Source: CAD feature listing. Evaluate the final solid. Frame: model axes, mm. Give positions to 0.01 mm unless a question says otherwise; leave off trailing zeros. Loops run counter-clockwise (first coordinate to the right, second up) from the corner with the lowest first, then second, coordinate; pieces in that order, holes last. Notation, with made-up numbers: M 39.25,9 L 58.25,9 A25 cw 58.25,39 Z; hole C 23.25,75.5 d1. An arc over 180 degrees is marked long. Put each result on its own line as item: value.
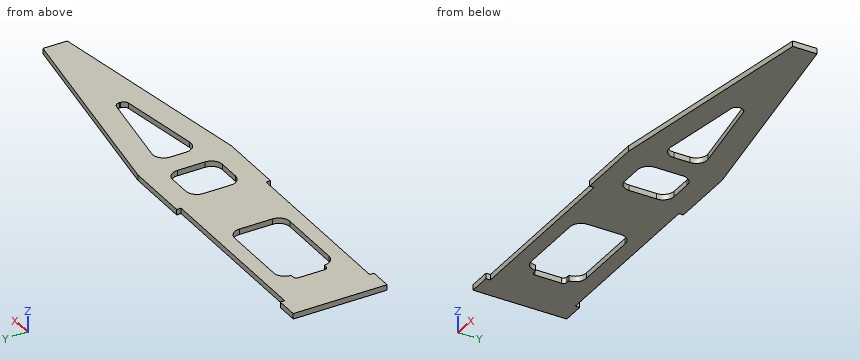
from build123d import *

# Parameters (mm, degrees)
GRUNDPLATTE_DEPTH                  = 5
SCHNITT_LINEAR_AUSTRAGEN1_DEPTH    = 443.076068115
VERRUNDUNG1_R                      = 10
SKIZZE3_W                          = 160
SKIZZE3_H                          = 4
AUSSCHNITT_FL_CHENAUFDOPPLER_DEPTH = 443.076068115
SKIZZE4_W                          = 40
SKIZZE4_H                          = 45
AUSSCHNITT_GEWICHT_DEPTH           = 443.076068115
VERRUNDUNG2_R                      = 10
VERRUNDUNG3_R                      = 5
VERRUNDUNG4_R                      = 3


with BuildPart() as part:
    # Skizze1 → Grundplatte (new body)
    with BuildSketch(Plane.XY):
        Polygon((0, 42.5), (0, -42.5), (240, -42.5), (440, -11), (440, 11), (240, 42.5), align=None)
    extrude(amount=GRUNDPLATTE_DEPTH)

    # Skizze2 → Schnitt-Linear austragen1 (cut, through all)
    with BuildSketch(Plane.XY.offset(5)):
        Polygon((130, 25), (50, 25), (50, 15), (44, 15), (44, -15), (50, -15), (50, -25), (130, -25), align=None)
    extrude(amount=-SCHNITT_LINEAR_AUSTRAGEN1_DEPTH, mode=Mode.SUBTRACT)

    # Verrundung1
    verrundung1_edges = [part.edges().sort_by_distance(p)[0] for p in [
        (130, 25, 2.5),
        (130, -25, 2.5),
        (50, 25, 2.5),
        (50, -25, 2.5),
    ]]
    fillet(verrundung1_edges, radius=VERRUNDUNG1_R - 0.0001)  # a hair under: the kernel refuses the full size

    # Skizze3 → Ausschnitt_Flächenaufdoppler (cut, through all)
    with BuildSketch(Plane.XY.offset(5)):
        with Locations((100, 40.5)):
            Rectangle(SKIZZE3_W, SKIZZE3_H)
        with Locations((100, -40.5)):
            Rectangle(SKIZZE3_W, SKIZZE3_H)
    extrude(amount=-AUSSCHNITT_FL_CHENAUFDOPPLER_DEPTH, mode=Mode.SUBTRACT)

    # Skizze4 → Ausschnitt Gewicht (cut, through all)
    with BuildSketch(Plane.XY.offset(5)):
        with Locations((210, 0)):
            Rectangle(SKIZZE4_W, SKIZZE4_H)
        Polygon((250, -19), (250, 19), (340, 4.825), (340, -4.825), align=None)
    extrude(amount=-AUSSCHNITT_GEWICHT_DEPTH, mode=Mode.SUBTRACT)

    # Verrundung2
    verrundung2_edges = [part.edges().sort_by_distance(p)[0] for p in [
        (190, 22.5, 2.5),
        (230, 22.5, 2.5),
        (230, -22.5, 2.5),
        (190, -22.5, 2.5),
        (250, -19, 2.5),
        (250, 19, 2.5),
    ]]
    fillet(verrundung2_edges, radius=VERRUNDUNG2_R)

    # Verrundung3
    verrundung3_edges = [part.edges().sort_by_distance(p)[0] for p in [
        (340, -4.825, 2.5),
        (340, 4.825, 2.5),
    ]]
    fillet(verrundung3_edges, radius=VERRUNDUNG3_R)

    # Verrundung4
    verrundung4_edges = [part.edges().sort_by_distance(p)[0] for p in [
        (44, -15, 2.5),
        (44, 15, 2.5),
    ]]
    fillet(verrundung4_edges, radius=VERRUNDUNG4_R)


solid = part.part
1. Section query A-A (x = 114). Output: boundary loops of the cut face in (y, z).
Found:
outline: M -38.5,0 L -25,0 L -25,5 L -38.5,5 Z; M 25,0 L 38.5,0 L 38.5,5 L 25,5 Z
2. Section query D-D (x = 388). Output: boundary loops of the cut face in (y, z), plus the area to 3 significant figures.
Found:
outline: M -19.19,0 L 19.19,0 L 19.19,5 L -19.19,5 Z
area: 192 mm^2
3. Section query C-C (x = 210). Output: boundary loops of the cut face in (y, z).
Found:
outline: M -42.5,0 L -22.5,0 L -22.5,5 L -42.5,5 Z; M 22.5,0 L 42.5,0 L 42.5,5 L 22.5,5 Z
4. Section query B-B (z = 2.1). State how many separate pieces and enclosed holes the cut face has, plus the area to 3 significant figures.
Found:
separate pieces: 1
enclosed holes: 3
area: 21,900 mm^2
5. Contact query for a flat-ended pin moving along its axis: P1, Ø2.5, axis at x = 48, z = 2.5, coming from the -Y side. Output: stop coordinate, or through.
Found:
P1: y = -38.5
6. Material intervals for line 1 (X direction, y = 0, z = 1.4); line 2 (Y direction, x = 80, z = 2.45); line 3 (X direction, y = 3, z = 1.4), sorted ascending. Write a range as from..to.
Found:
line 1: 0..44, 130..190, 230..250, 340..440
line 2: -38.5..-25, 25..38.5
line 3: 0..44, 130..190, 230..250, 339.36..440
